Could you check a few things on this model? Use its own coordinates, in mm. A direction names the side the tool comes from. Round coordinates to 2 decimals unless told otherwise and drop trailing zeros.
from build123d import *

# Parameters (mm, degrees)
SKETCH1_R                 = 114.3
BOSS_EXTRUDE1_DEPTH       = 23.8125
SKETCH2_R                 = 9.525
BOLTHOLE_DEPTH            = 164.389152505
BOLTHOLEPATTERN_COUNT     = 8
SKETCH5_OUTSIDE_W         = 295.434
SKETCH5_OUTSIDE_H         = 295.434
SKETCH5_OUTSIDE_R         = 78.58125
RAISED_FACE_DEPTH         = 1.5875
SKETCH8_R                 = 67.4624
WELD_NECK_120_DRAFT_DEPTH = 52.3875
WELD_NECK_120_DRAFT_TAPER = 30
WELD_NECK_END_REACH       = 180.705
SKETCH9_R                 = 57.15
WELD_NECK_CHAMFER1_SIZE   = 3.401023409
WELD_NECK_CHAMFER1_SIZE2  = 4.4323
SKETCH7_R                 = 51.1302
BORE_DEPTH                = 179.704840449
FILLET2_R                 = 1.5875
FILLET3_R                 = 1.5875


with BuildPart() as part:
    # Sketch1 → Boss-Extrude1 (new body)
    with BuildSketch(Plane.XY):
        Circle(SKETCH1_R)
    extrude(amount=BOSS_EXTRUDE1_DEPTH)

    # Sketch2 → BoltHole (cut, through all)
    with BuildSketch(Plane.XY):
        with Locations((36.450596933, 87.999525472)):
            Circle(SKETCH2_R)
    bolthole = extrude(amount=BOLTHOLE_DEPTH, mode=Mode.SUBTRACT)

    # BoltHolePattern: BoltHole ×8 about axis
    boltholepattern_axis = Axis((0, 0, 0), (0, 0, 1))
    for i in range(1, BOLTHOLEPATTERN_COUNT):
        add(bolthole.rotate(boltholepattern_axis, i * 360 / BOLTHOLEPATTERN_COUNT), mode=Mode.SUBTRACT)

    # Sketch5 outside → Raised Face (cut)
    with BuildSketch(Plane(origin=(0, 0, 0), x_dir=(-1, 0, 0), z_dir=(0, 0, -1))):
        Rectangle(SKETCH5_OUTSIDE_W, SKETCH5_OUTSIDE_H)
        Circle(SKETCH5_OUTSIDE_R, mode=Mode.SUBTRACT)
    extrude(amount=-RAISED_FACE_DEPTH, mode=Mode.SUBTRACT)

    # Sketch8 → Weld Neck 120 Draft (add)
    with BuildSketch(Plane.XY.offset(23.8125)):
        Circle(SKETCH8_R)
    extrude(amount=WELD_NECK_120_DRAFT_DEPTH, taper=WELD_NECK_120_DRAFT_TAPER)

    # Sketch9 → Weld Neck End (add, up to next)
    with BuildSketch(Plane.XY.offset(76.2), mode=Mode.PRIVATE) as weld_neck_end_sk1:
        Circle(SKETCH9_R)
    weld_neck_end_tool1 = extrude(weld_neck_end_sk1.sketch, amount=-WELD_NECK_END_REACH, mode=Mode.PRIVATE) - part.part
    add(weld_neck_end_tool1.solids().sort_by_distance((0, 0, 76.2))[0])

    # Weld Neck Chamfer1
    weld_neck_chamfer1_edges = [part.edges().sort_by_distance(p)[0] for p in [
        (-57.15, 0, 76.2),
    ]]
    weld_neck_chamfer1_side = [part.faces().sort_by_distance(p)[0] for p in [
        (-57.15, 0, 58.937050374),
    ]]
    chamfer(weld_neck_chamfer1_edges, length=WELD_NECK_CHAMFER1_SIZE, length2=WELD_NECK_CHAMFER1_SIZE2, reference=weld_neck_chamfer1_side[0])

    # Sketch7 → Bore (cut, through all)
    with BuildSketch(Plane.XY):
        with Locations(Location((0, 0, 0), (0, 0, 180))):
            Circle(SKETCH7_R)
    extrude(amount=BORE_DEPTH, mode=Mode.SUBTRACT)

    # Fillet2
    fillet2_edges = [part.edges().sort_by_distance(p)[0] for p in [
        (-114.3, 0, 23.8125),
        (-114.3, 0, 1.5875),
    ]]
    fillet(fillet2_edges, radius=FILLET2_R)

    # Fillet3
    fillet3_edges = [part.edges().sort_by_distance(p)[0] for p in [
        (78.58125, 0, 1.5875),
    ]]
    fillet(fillet3_edges, radius=FILLET3_R - 0.0001)  # a hair under: the kernel refuses the full size


solid = part.part
Item 1: We'd pull the mould along X, two halves only. Please class faces 4 (the flat face through (49, -49, 23.812)), 5 (the conical face through (-6.891, 52.482, 76.035)), 6 (the cylindrical face through (-97.3, -38.5, 12.5)): released by +X, released by -X, zero draft, split by the parting line, or undercut.
Results list:
face 4: zero draft
face 5: split by the parting line
face 6: undercut
Item 2: If I drill on line 1 along Y through (x, z) = (83, 15); line 2 along Z through (x, y) = (-56, 67); line 3 along Y through (x, z) = (4, 20), over which ranges is the centre line in solid material (lowest first)?
Results list:
line 1: y = -78.58 to -44.56, -28.34 to 28.34, 44.56 to 78.58
line 2: z = 1.59 to 23.81
line 3: y = -114.23 to -50.97, 50.97 to 114.23
Item 3: If we section it at C-C, the plane z = 11: Count the separate pieces of the cut face and the enclosed holes in it, then the cut area to 4 significant figures.
Results list:
separate pieces: 1
enclosed holes: 9
area: 30,550 mm2
Item 4: For faces 1 (the cylindrical face through (-57.095, 2.513, 57.454)), 2 (the cylindrical face through (-78.7, 34.39, 12.54)), 3 (the flat face through (77, -23, 1.588)), which set-ups out of +Z, -Z, +X, -X, +Y, -Y let a thin tool reach every point of the face, with its end or its side?
Results list:
face 1: +Z
face 2: +Z, -Z
face 3: -Z
Item 5: Will these pins go through, and if not, where does the flat tip stop? pin 1 (15 mm diameter, centred on x = 88, y = -36.45, fed in from +Z); pin 2 (25 mm diameter, centred on x = 36.45, y = 88, fed in from -Z); pin 3 (4 mm diameter, centred on x = -40.5, z = 10.5, fed in from +Y); pin 4 (3 mm diameter, centred on x = -12.5, z = 48.5, fed in from -Y).
Results list:
pin 1: passes through
pin 2: stops at z = 1.59
pin 3: stops at y = 107.62
pin 4: stops at y = -56.08
